```python
from build123d import *

# Parameters (mm, degrees)
BOSS_EXTRUDE1_DEPTH      = 14.25
BOSS_EXTRUDE1_DEPTH_BACK = 14.25
SKETCH2_R                = 5
BOSS_EXTRUDE2_DEPTH      = 7
SKETCH3_R                = 2.25
CUT_EXTRUDE1_DEPTH       = 1.5
SKETCH4_R                = 1.5
CUT_EXTRUDE2_DEPTH       = 10.5
SKETCH5_R                = 3.25
CUT_EXTRUDE3_DEPTH       = 32.5


with BuildPart() as part:
    # Sketch1 → Boss-Extrude1 (new body, two sides)
    with BuildSketch(Plane(origin=(0, 0, 0), x_dir=(1, 0, 0), z_dir=(0, 1, 0))) as boss_extrude1_sk:
        with BuildLine():
            Line((-14.25, 9.25), (-14.25, -12.25))
            Line((-14.25, -12.25), (-11.25, -12.25))
            Line((-11.25, -12.25), (-11.25, 8.25))
            Line((-11.25, 8.25), (11.25, 8.25))
            Line((11.25, 8.25), (11.25, -12.25))
            Line((11.25, -12.25), (14.25, -12.25))
            Line((14.25, -12.25), (14.25, 9.25))
            ThreePointArc((14.25, 9.25), (13.371320344, 11.371320344), (11.25, 12.25))
            Line((11.25, 12.25), (-11.25, 12.25))
            ThreePointArc((-11.25, 12.25), (-13.371320344, 11.371320344), (-14.25, 9.25))
        make_face()
    extrude(amount=BOSS_EXTRUDE1_DEPTH)
    extrude(boss_extrude1_sk.sketch, amount=-BOSS_EXTRUDE1_DEPTH_BACK)

    # Sketch2 → Boss-Extrude2 (add)
    with BuildSketch(Plane(origin=(0, 0, -12.25), x_dir=(-1, 0, 0), z_dir=(0, 0, -1))):
        Circle(SKETCH2_R)
    extrude(amount=BOSS_EXTRUDE2_DEPTH)

    # Sketch3 → Cut-Extrude1 (cut)
    with BuildSketch(Plane(origin=(0, 0, -19.25), x_dir=(-1, 0, 0), z_dir=(0, 0, -1))):
        Circle(SKETCH3_R)
    extrude(amount=-CUT_EXTRUDE1_DEPTH, mode=Mode.SUBTRACT)

    # Sketch4 → Cut-Extrude2 (cut)
    with BuildSketch(Plane(origin=(0, 0, -17.75), x_dir=(-1, 0, 0), z_dir=(0, 0, -1))):
        Circle(SKETCH4_R)
    extrude(amount=-CUT_EXTRUDE2_DEPTH, mode=Mode.SUBTRACT)

    # Sketch5 → Cut-Extrude3 (cut)
    with BuildSketch(Plane(origin=(14.25, 0, 0), x_dir=(0, 0, -1), z_dir=(1, 0, 0))):
        with Locations((-2, 0)):
            Circle(SKETCH5_R)
    extrude(amount=-CUT_EXTRUDE3_DEPTH, mode=Mode.SUBTRACT)


solid = part.part
```
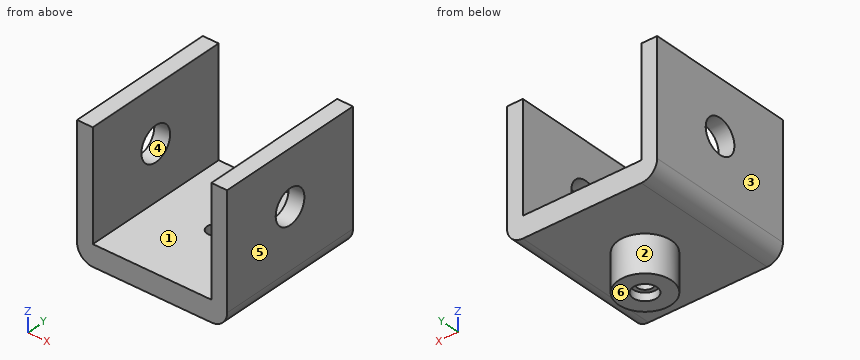
The listing builds one solid part. Answer for the finished solid, in the listing's coordinates (mm). Face numbers are marked on the shaded views. A direction names the side the tool comes from. Coordinates: 2 decimals unless noted, no trailing zeros. Write each loop counter-clockwise with the first axis right and the second up, starting at its lowest first coordinate (ties: lowest second). Pieces come first, ordered by that corner, then holes. Notation, with made-up numbers: (53.5, 50) - (78.5, 50) arc R35 ccw to (78.5, 83) - close; hole circle Ø1 at (0, 69). An arc over 180 degrees is marked (long way). Return JSON: item names as keys, results as strings. Group by question number.
1. A cutting plane is placed at A-A, the plane z = 2. Determine the outline of the cut face in (x, y), plus the area to 3 significant figures.
2. Straight lines are drawn through the part: L1, parallel to Y at x = 0, z = -18.9; L2, parallel to Y at x = -12.95, z = 2; L3, parallel to X at y = -7.75, z = 1.5. For each, find the intervals that lie inside material, in ascending order.
3. A cutting plane is placed at D-D, the plane z = -5. Determine the outline of the cut face in (x, y).
4. Determine the mould class of the marked faces 4, 5 and 6 for opening direction Z: released by +Z, released by -Z, zero draft, split by the parting line, or undercut.
5. A cutting plane is placed at B-B, the plane x = 0. Determine the outline of the cut face in (y, z), plus the area to 3 significant figures.
6. Which of the six approach directions +Z, -Z, +X, -X, +Y, -Y give full straight-line access (tool end or side, diameter ignored) to the marked faces 1, 2 and 3?
7. Given pin 1 (4 mm diameter, centred on x = -2.5, y = 3.5, fed in from +Z); pin 2 (2.5 mm diameter, centred on x = 0, y = 0, fed in from -Z); pin 3 (2 mm diameter, centred on y = 1.5, z = -10.5, fed in from +X); pin 4 (2 mm diameter, centred on x = -1, y = 7.5, fed in from -Z), each flat-ended and moving along its own axis, determine where each tip first touches the part or whether it passes through.
8. A cutting plane is placed at C-C, the plane y = 0. Give the number of separate pieces and of enclosed holes in the cut face, plus the area to 3 significant figures.
Ans:
{
 "1": {"outline": "(-14.25, -14.25) - (-11.25, -14.25) - (-11.25, -3.25) - (-14.25, -3.25) - close; (-14.25, 3.25) - (-11.25, 3.25) - (-11.25, 14.25) - (-14.25, 14.25) - close; (11.25, -14.25) - (14.25, -14.25) - (14.25, -3.25) - (11.25, -3.25) - close; (11.25, 3.25) - (14.25, 3.25) - (14.25, 14.25) - (11.25, 14.25) - close", "area": "132 mm²"},
 "2": {"L1": "-5 to -2.25, 2.25 to 5", "L2": "-14.25 to -3.25, 3.25 to 14.25", "L3": "-14.25 to -11.25, 11.25 to 14.25"},
 "3": {"outline": "(-14.25, -14.25) - (-11.25, -14.25) - (-11.25, 14.25) - (-14.25, 14.25) - close; (11.25, -14.25) - (14.25, -14.25) - (14.25, 14.25) - (11.25, 14.25) - close"},
 "4": {"face 4": "undercut", "face 5": "zero draft", "face 6": "released by -Z"},
 "5": {"outline": "(-14.25, -12.25) - (-5, -12.25) - (-5, -19.25) - (-2.25, -19.25) - (-2.25, -17.75) - (-1.5, -17.75) - (-1.5, -8.25) - (-14.25, -8.25) - close; (1.5, -17.75) - (2.25, -17.75) - (2.25, -19.25) - (5, -19.25) - (5, -12.25) - (14.25, -12.25) - (14.25, -8.25) - (1.5, -8.25) - close", "area": "149 mm²"},
 "6": {"face 1": "+Z, +Y, -Y", "face 2": "-Z", "face 3": "+Z, -Z, -X, +Y, -Y"},
 "7": {"pin 1": "z = -8.25", "pin 2": "through", "pin 3": "x = 14.24", "pin 4": "z = -12.25"},
 "8": {"separate pieces": "4", "enclosed holes": "0", "area": "229 mm²"}
}
